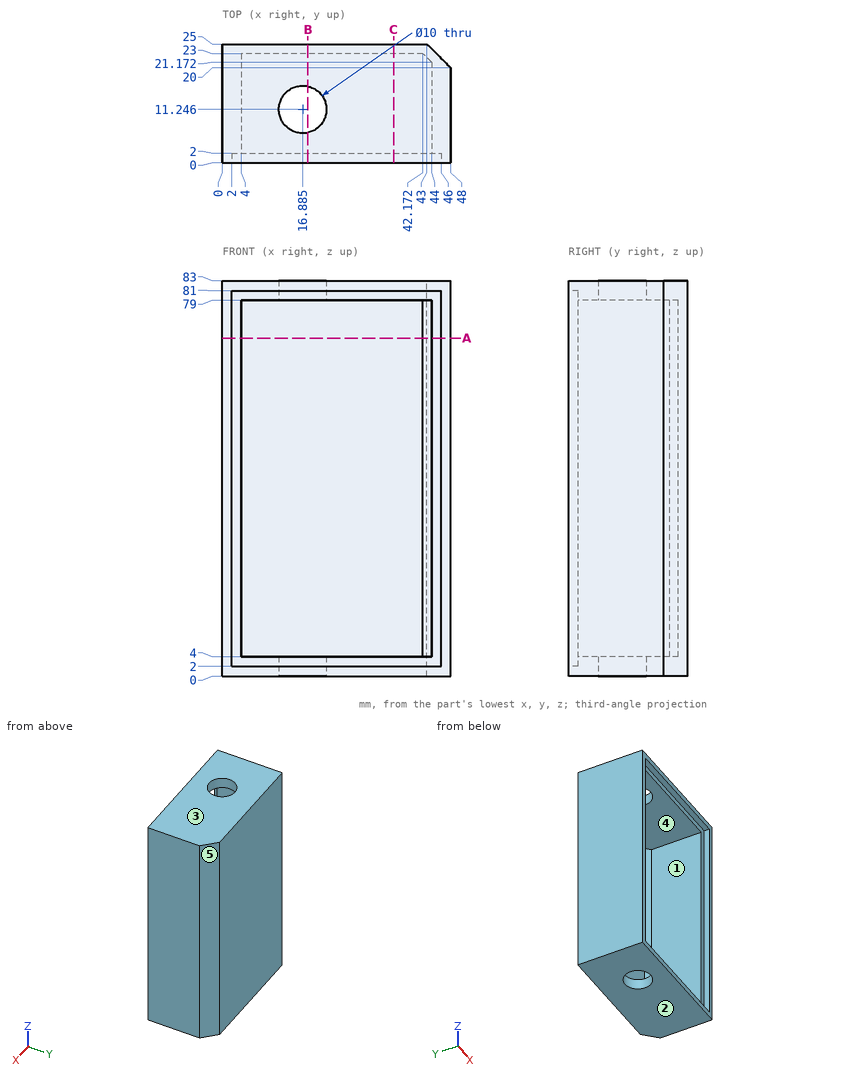
For this review, use the dimensioned drawing (mm, ordinates from the lowest corner) and the shaded views. A direction names the side the tool comes from. Give positions to 0.01 mm unless a question says otherwise; leave off trailing zeros. Order: outer loops, then holes, each group sorted by start corner. A loop starts at its lowest first (then second) coordinate and runs counter-clockwise, first axis right, second up. Notation, with made-up numbers: M -25.5,43 L -17.5,43 A22 ccw -17.5,74 Z; hole C -31.75,82.5 d4. An arc over 180 degrees is marked long. Use one line per item in the form item = value. Start each with the question number.
Item 1: The part is to be moulded in two halves that separate along Z. For the marked faces 1, 2 and 3, say which applies: pulls with the +Z half, pulls with the -Z half, needs draft (parallel to the pull), parting line crosses it, or undercut.
Item 2: For the marked faces 4 and 5, list the 3-axis set-ups (+Z, -Z, +X, -X, +Y, -Y) from which the entire face can be reached by the end or side of a thin tool; tool diameter is ignored.
Item 3: We need section B-B on x = 18. Give the boundary of the cut face in (y, z).
Item 4: We need section C-C on x = 36. Give the boundary of the cut face in (y, z), plus the area to 3 significant figures.
Item 5: Insertion check: pin 1 Ø22 at (x, z) = (18.5, 29) entering from -Y. The pin has a flat end and moves straight along its axis. Give the tip position at first contact, or say it passes through.
Item 6: We need section A-A on z = 71. Give the boundary of the cut face in (x, y).
Item 7: To check wall thickness, follow line 1 along Z through (x, y) = (8, 3); line 2 along X through (y, z) = (8.75, 57); line 3 along Y through (x, z) = (39, 5). State the ranges of each line that lie inside material, in increasing order. Write a range as from..to.
Completed:
q1.face_1 = undercut
q1.face_2 = pulls with the -Z half
q1.face_3 = pulls with the +Z half
q2.face_4 = -Y
q2.face_5 = +Z, -Z, +X, +Y
q3.outline = M 0,0 L 6.37,0 L 6.37,4 L 2,4 L 2,2 L 0,2 Z; M 0,81 L 2,81 L 2,79 L 6.37,79 L 6.37,83 L 0,83 Z; M 16.12,0 L 25,0 L 25,83 L 16.12,83 L 16.12,79 L 23,79 L 23,4 L 16.12,4 Z
q4.outline = M 0,0 L 25,0 L 25,83 L 0,83 L 0,81 L 2,81 L 2,79 L 23,79 L 23,4 L 2,4 L 2,2 L 0,2 Z
q4.area = 342 mm²
q5.pin_1 = 23
q6.outline = M 0,0 L 2,0 L 2,2 L 4,2 L 4,23 L 42.17,23 L 44,21.17 L 44,2 L 46,2 L 46,0 L 48,0 L 48,20 L 43,25 L 0,25 Z
q7.line_1 = 0..4, 79..83
q7.line_2 = 0..4, 44..48
q7.line_3 = 23..25
